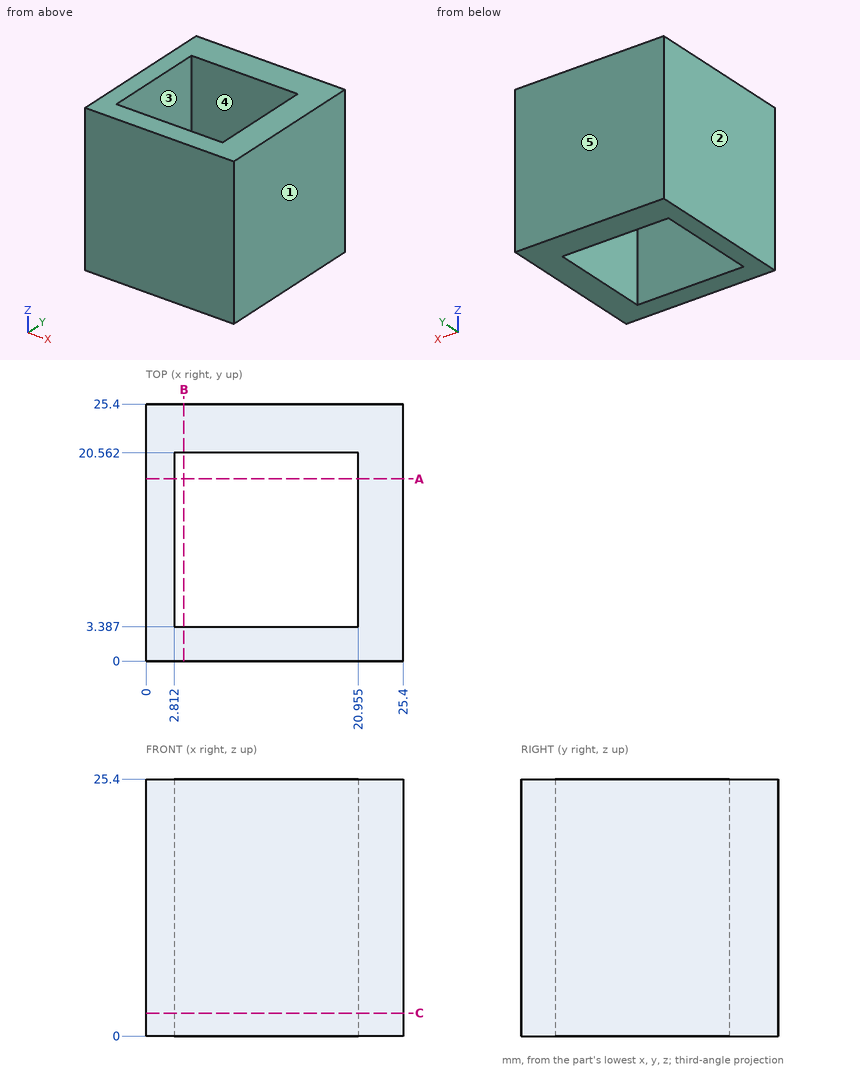
Answer from the drawing. Dimensions are ordinates in mm from the lowest x, y and z of the part. A direction names the side the tool comes from. Give positions to 0.01 mm unless a question says otherwise; leave off trailing zeros. Order: outer loops, then holes, each group sorted by start corner. A loop starts at its lowest first (then second) coordinate and runs counter-clockwise, first axis right, second up.
Item 1: The part is cut by section A-A, the plane y = 18. Give the vertices of the cut face in (x, z) (1 decimal), and give its area (3 significant figures).
From the geometry:
outline: (0, 0) - (2.8, 0) - (2.8, 25.4) - (0, 25.4) - close; (21, 0) - (25.4, 0) - (25.4, 25.4) - (21, 25.4) - close
area: 184 mm2
Item 2: Which of the six approach directions +Z, -Z, +X, -X, +Y, -Y give full straight-line access (tool end or side, diameter ignored) to the marked faces 4 and 5?
From the geometry:
face 4: +Z, -Z
face 5: +Z, -Z, +X, -X, +Y
Item 3: Given pin 1 Ø2 at (x, y) = (4, 11) entering from -Z, flat-ended and moving along its own axis, determine where the tip first touches the part or whether it passes through.
From the geometry:
pin 1: passes through
Item 4: For a pull along X with two mould halves and no side action, classify the marked faces 1, 2 and 3 as pulls with the +X half, pulls with the -X half, needs draft (parallel to the pull), parting line crosses it, or undercut.
From the geometry:
face 1: pulls with the +X half
face 2: pulls with the -X half
face 3: undercut
Item 5: Find the intervals of material crossed by probe 1 along X at (y, z) = (10.5, 19.75) (1 decimal); probe 2 along Y at (x, z) = (13.75, 13.75), in increasing order.
From the geometry:
probe 1: x = 0 to 2.8, 21 to 25.4
probe 2: y = 0 to 3.39, 20.56 to 25.4
Item 6: The part is cut by section B-B, the plane x = 3.75. Give the vertices of the cut face in (y, z), and give its area (3 significant figures).
From the geometry:
outline: (0, 0) - (3.39, 0) - (3.39, 25.4) - (0, 25.4) - close; (20.56, 0) - (25.4, 0) - (25.4, 25.4) - (20.56, 25.4) - close
area: 209 mm2
Item 7: The part is cut by section C-C, the plane z = 2.25. Give the vertices of the cut face in (x, y) (1 decimal).
From the geometry:
outline: (0, 0) - (25.4, 0) - (25.4, 25.4) - (0, 25.4) - close; hole (2.8, 3.4) - (21, 3.4) - (21, 20.6) - (2.8, 20.6) - close
